from build123d import *

# Parameters (mm, degrees)
F0_R     = 31
F1_DEPTH = 82
F2_R     = 27
F3_DEPTH = 78
F4_R     = 4
F5_DEPTH = 4
F7_R     = 4
F8_DEPTH = 4.2989402544


with BuildPart() as f1:
    # F0 (on Top) → F1 (new body)
    with BuildSketch(Plane.XY):
        Circle(F0_R)
    extrude(amount=F1_DEPTH)

    # F2 (on face) → F3 (cut)
    with BuildSketch(Plane.XY.offset(82)):
        Circle(F2_R)
    extrude(amount=-F3_DEPTH, mode=Mode.SUBTRACT)

    # F4 (on face) → F5 (cut, through all)
    with BuildSketch(Plane(origin=(0, 0, 0), x_dir=(1, 0, 0), z_dir=(0, 0, -1))):
        Circle(F4_R)
    extrude(amount=-F5_DEPTH, mode=Mode.SUBTRACT)

    # F7 (on offset) → F8 (cut, through all)
    with BuildSketch(Plane.YZ.offset(31)):
        with Locations((0, 73)):
            Circle(F7_R)
    extrude(amount=-F8_DEPTH, mode=Mode.SUBTRACT)


solid = f1.part
Could you check a few things on this model? Use its own coordinates, in mm. A direction names the side the tool comes from. Give positions to 0.01 mm unless a question says otherwise; leave off trailing zeros. Order: outer loops, then holes, each group sorted by start corner. A loop starts at its lowest first (then second) coordinate and runs counter-clockwise, first axis right, second up.
1. Suppose I cut it at B-B (y = 0). Write out the boundary of the cut face in (x, z).
Answers below:
outline: (-31, 0) - (-4, 0) - (-4, 4) - (-27, 4) - (-27, 82) - (-31, 82) - close; (4, 0) - (31, 0) - (31, 69) - (27, 69) - (27, 4) - (4, 4) - close; (27, 77) - (31, 77) - (31, 82) - (27, 82) - close
2. I need wall thicknesses on L1, parallel to Y at x = 0, z = 3; L2, parallel to Y at x = 0, z = 39; L3, parallel to X at y = 10.5, z = 30. Which ranges of each line are inside material? Lowest first, please.
Answers below:
L1: y = -31 to -4, 4 to 31
L2: y = -31 to -27, 27 to 31
L3: x = -29.17 to -24.87, 24.87 to 29.17
3. Suppose I cut it at A-A (x = 0). Write out the boundary of the cut face in (y, z).
Answers below:
outline: (-31, 0) - (-4, 0) - (-4, 4) - (-27, 4) - (-27, 82) - (-31, 82) - close; (4, 0) - (31, 0) - (31, 82) - (27, 82) - (27, 4) - (4, 4) - close
4. Thinking about a two-plate mould opening in X: for faces 1 (the cylindrical face through (-4.036, 30.736, 40.426)), 2 (the flat face through (2, 28, 82)), 3 (the flat face through (6, 0, 4)), 4 (the cylindrical face through (-0.867, 3.905, 1.972)), which applies, +X half, -X half, draft (parallel to the pull), parting line (faces both ways), or undercut?
Answers below:
face 1: parting line
face 2: draft
face 3: undercut
face 4: undercut
5. Suppose I cut it at D-D (y = 16). Write out the boundary of the cut face in (x, z), plus the area to 3 significant figures.
Answers below:
outline: (-26.55, 0) - (26.55, 0) - (26.55, 82) - (21.75, 82) - (21.75, 4) - (-21.75, 4) - (-21.75, 82) - (-26.55, 82) - close
area: 962 mm2
6. Suppose I cut it at C-C (z = 25). Write out the boundary of the cut face in (x, y).
Answers below:
outline: circle Ø62 at (0, 0); hole circle Ø54 at (0, 0)
7. For pin 1 (5 mm diameter, centred on x = -8, y = -15.5, fed in from +Z); pin 2 (3 mm diameter, centred on y = -5, z = 53, fed in from +X); pin 3 (4 mm diameter, centred on y = -22.5, z = 73.5, fed in from +X), each with a flat end and sliding along its axis, tell me the tip position at first contact or that it passes through.
Answers below:
pin 1: stops at z = 4
pin 2: stops at x = 30.8
pin 3: stops at x = 23.25
8. Which directions (+Z, -Z, +X, -X, +Y, -Y) give clear straight access to the entire face, cutting with the end or side of a thin tool? Please do faces 5 (the flat face through (0, -6, 0)), 6 (the cylindrical face through (-5.85, -26.36, 43.55)), 7 (the cylindrical face through (29, -4, 73)).
Answers below:
face 5: -Z, +X, -X, +Y, -Y
face 6: +Z
face 7: +X
